```python
from build123d import *

# Parameters (mm, degrees)
ESQUISSE1_R             = 26
ESQUISSE1_R_2           = 2
BOSS_EXTRU_1_DEPTH      = 1
ESQUISSE1_3_R           = 26
BOSS_EXTRU_2_DEPTH      = 25
ESQUISSE2_R             = 25
ENL_V_MAT_EXTRU_1_DEPTH = 10


with BuildPart() as part:
    # Esquisse1 → Boss.-Extru.1 (new body)
    # profile 1 of 3: a face of its own
    with BuildSketch(Plane.XY):
        Circle(ESQUISSE1_R)
    # profile 2 of 3: a face of its own
    with BuildSketch(Plane.XY):
        with BuildLine():
            ThreePointArc((-25.057692308, -6.936285477), (-26, 0), (-25.057692308, 6.936285477))
            ThreePointArc((-25.057692308, 6.936285477), (-33, 0), (-25.057692308, -6.936285477))
        make_face()
        with Locations((-30, 0)):
            Circle(ESQUISSE1_R_2, mode=Mode.SUBTRACT)
    # profile 3 of 3: a face of its own
    with BuildSketch(Plane.XY):
        with BuildLine():
            ThreePointArc((25.057692308, 6.936285477), (25.763346056, 3.5), (26, 0))
            ThreePointArc((26, 0), (25.763346056, -3.5), (25.057692308, -6.936285477))
            ThreePointArc((25.057692308, -6.936285477), (33, 0), (25.057692308, 6.936285477))
        make_face()
        with Locations((30, 0)):
            Circle(ESQUISSE1_R_2, mode=Mode.SUBTRACT)
    extrude(amount=BOSS_EXTRU_1_DEPTH)

    # Esquisse1_3 → Boss.-Extru.2 (add)
    with BuildSketch(Plane.XY):
        with Locations(Location((0, 0, 0), (0, 0, 164.52723992))):
            Circle(ESQUISSE1_3_R)
    extrude(amount=BOSS_EXTRU_2_DEPTH)

    # Esquisse2 → Enl_v. mat.-Extru.1 (cut)
    with BuildSketch(Plane.XY.offset(25)):
        Circle(ESQUISSE2_R)
    extrude(amount=-ENL_V_MAT_EXTRU_1_DEPTH, mode=Mode.SUBTRACT)


solid = part.part
```
Could you check a few things on this model? Use its own coordinates, in mm. Coordinates: 2 decimals unless noted, no trailing zeros. Order: outer loops, then holes, each group sorted by start corner. A loop starts at its lowest first (then second) coordinate and runs counter-clockwise, first axis right, second up. Notation, with made-up numbers: M 38,38 L 47,38 A27 ccw 47,73 Z; hole C 70,55.5 d2. An arc over 180 degrees is marked long. Use one line per item in the form item = value. Start each with the question number.
1. Please list where these lines run through material, in increasing order: line 1 (Y direction, x = 0, z = 19.5); line 2 (Z direction, x = -15.5, y = 19); line 3 (X direction, y = -18.5, z = 17.75).
2. Suppose I cut it at B-B on x = -30. Write out the boundary of the cut face in (y, z), then the cut area to 3 significant figures.
3. For pin 1 (4 mm diameter, centred on x = -3.5, z = 7, fed in from -Y); pin 2 (10 mm diameter, centred on y = -12, z = 9.5, fed in from -X); pin 3 (8 mm diameter, centred on x = 13, z = 17.5, fed in from +Y), each with a flat end and sliding along its axis, tell me the tip position at first contact or that it passes through.
4. Suppose I cut it at A-A on y = 0. Write out the boundary of the cut face in (x, z).
5. Suppose I cut it at C-C on y = -11. Write out the boundary of the cut face in (x, z).
6. Suppose I cut it at D-D on x = -18. Write out the boundary of the cut face in (y, z), then the cut area to 3 significant figures.
7. We'd pull the mould along X, two halves only. Please class faces 1 (the flat face through (0, 0, 15)), 2 (the cylindrical face through (23.846, 7.509, 20.07)), 3 (the flat face through (0, 0, 0)): +X half, -X half, draft (parallel to the pull), parting line (faces both ways), or undercut.
Geometry says:
q1.line_1 = -26 to -25, 25 to 26
q1.line_2 = 0 to 15
q1.line_3 = -18.27 to -16.82, 16.82 to 18.27
q2.outline = M -5.74,0 L -2,0 L -2,1 L -5.74,1 Z; M 2,0 L 5.74,0 L 5.74,1 L 2,1 Z
q2.area = 7.49 mm^2
q3.pin_1 = -25.96
q3.pin_2 = -25.04
q3.pin_3 = 24.39
q4.outline = M -33,0 L -32,0 L -32,1 L -33,1 Z; M -28,0 L 28,0 L 28,1 L 26,1 L 26,25 L 25,25 L 25,15 L -25,15 L -25,25 L -26,25 L -26,1 L -28,1 Z; M 32,0 L 33,0 L 33,1 L 32,1 Z
q5.outline = M -23.56,0 L 23.56,0 L 23.56,25 L 22.45,25 L 22.45,15 L -22.45,15 L -22.45,25 L -23.56,25 Z
q6.outline = M -18.76,0 L 18.76,0 L 18.76,25 L 17.35,25 L 17.35,15 L -17.35,15 L -17.35,25 L -18.76,25 Z
q6.area = 591 mm^2
q7.face_1 = undercut
q7.face_2 = undercut
q7.face_3 = draft
